Part print with two shaded views. Sizes in mm from the minimum x, y, z corner. Give positions to 0.01 mm unless a question says otherwise; leave off trailing zeros. Write each loop counter-clockwise with the first axis right and the second up, starting at its lowest first coordinate (ties: lowest second). Pieces come first, ordered by that corner, then holes. Notation, with made-up numbers: M 85.5,31 L 132.5,31 A30 cw 132.5,68 Z; hole C 28,-1.75 d7. An arc over 180 degrees is marked long. One line per item, written item: value. Start each with the question number.
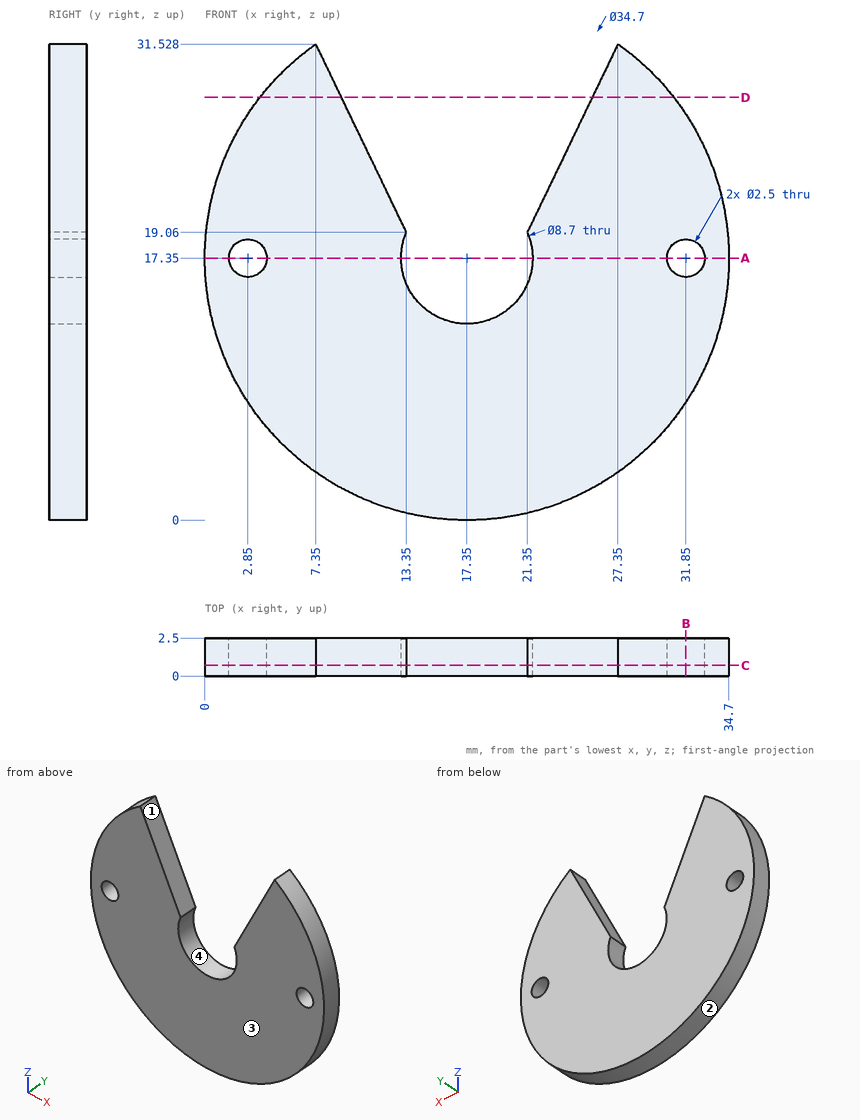
1) Drop a flat-ended pin along its axis: P1, Ø6, axis at x = 10.5, z = 8, coming from the -Y side. Give the stop position or say it passes through.
2) Band-saw the part on D-D (z = 28). List the corners of the cut face in (x, y).
3) Band-saw the part on B-B (x = 31.85). List the corners of the cut face in (y, z).
4) Probe line 1 along X through (y, z) = (0.7, 17.35); line 2 along X through (y, z) = (0.45, 18); line 3 along Z through (x, y) = (17.35, 1.65). List the from-to ranges inside material, lowest first. Write a range as from..to.
5) Band-saw the part on A-A (z = 17.35). List the corners of the cut face in (x, y).
6) Band-saw the part on C-C (y = 0.7). List the corners of the cut face in (x, z).
7) Mould opens along Z. For the marked faces 1, 2, 3 and 4 say: released by +Z, released by -Z, zero draft, split by the parting line, or undercut.
Model answer:
1. P1: stops at y = 0
2. outline: M 3.65,0 L 9.05,0 L 9.05,2.5 L 3.65,2.5 Z; M 25.65,0 L 31.05,0 L 31.05,2.5 L 25.65,2.5 Z
3. outline: M 0,7.82 L 2.5,7.82 L 2.5,16.1 L 0,16.1 Z; M 0,18.6 L 2.5,18.6 L 2.5,26.88 L 0,26.88 Z
4. line 1: x = 0..1.6, 4.1..13, 21.7..30.6, 33.1..34.7
4. line 2: x = 0.01..1.78, 3.92..13.05, 21.65..30.78, 32.92..34.69
4. line 3: z = 0..13
5. outline: M 0,0 L 1.6,0 L 1.6,2.5 L 0,2.5 Z; M 4.1,0 L 13,0 L 13,2.5 L 4.1,2.5 Z; M 21.7,0 L 30.6,0 L 30.6,2.5 L 21.7,2.5 Z; M 33.1,0 L 34.7,0 L 34.7,2.5 L 33.1,2.5 Z
6. outline: M 7.35,31.53 A17.35 ccw long 27.35,31.53 L 21.35,19.06 A4.35 cw long 13.35,19.06 Z; hole C 2.85,17.35 d2.5; hole C 31.85,17.35 d2.5
7. face 1: released by +Z
7. face 2: split by the parting line
7. face 3: zero draft
7. face 4: undercut
